Build history of the part. All positions in model axes, mm. A direction names the side the tool comes from. Round coordinates to 2 decimals unless told otherwise and drop trailing zeros. Write each loop counter-clockwise with the first axis right and the second up, starting at its lowest first coordinate (ties: lowest second). Pieces come first, ordered by that corner, then holes. Notation, with made-up numbers: (39, 25) -> (98, 25) arc R7 cw to (98, 29) -> close; hole circle Ø9 at (66.5, 13). An arc over 180 degrees is marked (long way). One line per question, with ' | ' between items.
from build123d import *

# Parameters (mm, degrees)
SKETCH002_R     = 6.5
SKETCH002_R_2   = 3
PAD_DEPTH       = 8
SKETCH003_R     = 7.7
POCKET_DEPTH    = 2
SKETCH004_R     = 3
POCKET001_DEPTH = 31
SKETCH005_R     = 2
PAD001_DEPTH    = 2


with BuildPart() as part:
    # Sketch002 → Pad (new body)
    with BuildSketch(Plane.XZ):
        with BuildLine():
            Line((-6.339746, 5), (6.339746, 5))
            ThreePointArc((25, 0), (17.58819, 9.659258), (6.339746, 5))
            Line((25, -14.5), (25, 0))
            Line((15, -14.5), (25, -14.5))
            Line((15, -10), (15, -14.5))
            ThreePointArc((6.339746, -5), (10, -8.660254), (15, -10))
            Line((-6.339746, -5), (6.339746, -5))
            ThreePointArc((-15, -10), (-10, -8.660254), (-6.339746, -5))
            Line((-15, -10), (-15, -14.5))
            Line((-25, -14.5), (-15, -14.5))
            Line((-25, 0), (-25, -14.5))
            ThreePointArc((-6.339746, 5), (-17.58819, 9.659258), (-25, 0))
        make_face()
        with Locations((-15, 0)):
            Circle(SKETCH002_R, mode=Mode.SUBTRACT)
        with Locations((15, 0)):
            Circle(SKETCH002_R, mode=Mode.SUBTRACT)
        Circle(SKETCH002_R_2, mode=Mode.SUBTRACT)
    extrude(amount=PAD_DEPTH)

    # Sketch003 (on Face16 of Pad) → Pocket (cut)
    with BuildSketch(Plane(origin=(0, 0, 0), x_dir=(1, 0, 0), z_dir=(0, 1, 0))):
        with Locations((-15, 0)):
            Circle(SKETCH003_R)
        with Locations((15, 0)):
            Circle(SKETCH003_R)
    extrude(amount=-POCKET_DEPTH, mode=Mode.SUBTRACT)

    # Sketch004 → Pocket001 (cut, symmetric)
    with BuildSketch(Plane.YZ):
        with Locations((-4, -10)):
            Circle(SKETCH004_R)
    extrude(amount=POCKET001_DEPTH, both=True, mode=Mode.SUBTRACT)

    # Sketch005 → Pad001 (join)
    with BuildSketch(Plane.XY.offset(-14.5)):
        with BuildLine():
            Line((-25, 0), (-15, 0))
            Line((-15, 0), (-15, 3.5))
            ThreePointArc((-15, 3.5), (-20, 8.5), (-25, 3.5))
            Line((-25, 0), (-25, 3.5))
        make_face()
        with Locations((-20, 3.5)):
            Circle(SKETCH005_R, mode=Mode.SUBTRACT)
        with BuildLine():
            Line((15, 0), (25, 0))
            Line((25, 0), (25, 3.5))
            ThreePointArc((25, 3.5), (20, 8.5), (15, 3.5))
            Line((15, 0), (15, 3.5))
        make_face()
        with Locations((20, 3.5)):
            Circle(SKETCH005_R, mode=Mode.SUBTRACT)
    extrude(amount=PAD001_DEPTH)


solid = part.part
(1) Mould opens along Z. For faces 1 (the flat face through (12, -2, 6)), 2 (the flat face through (20, 0, -14.5)), 3 (the cylindrical face through (18.002, 3.588, -13.514)) say: pulls with the +Z half, pulls with the -Z half, needs draft (parallel to the pull), parting line crosses it, or undercut.
Calculated:
face 1: undercut | face 2: pulls with the -Z half | face 3: needs draft
(2) 3-axis set-ups, long thin cutter, end or side, ignore diameter. For faces 4 (the cylindrical face through (-7, -4, -6)), 5 (the flat face through (18.8, 5.3, -12.5)), 6 (the flat face through (-18, -2, 6)), 7 (the flat face through (0, -4, 5)): which of +Z, -Z, +X, -X, +Y, -Y reach the whole face in a straight line?
Calculated:
face 4: -Z, +Y, -Y | face 5: +Z, +X, -X, +Y | face 6: +Y | face 7: +Z, +Y, -Y
(3) Wall check: line 1 (Y direction, x = -19.75, z = -10); line 2 (Y direction, x = -20, z = -13.45); line 3 (Z direction, x = -15.5, y = -4). Give the ranges that are in metal, low to high. Write a range as from..to.
Calculated:
line 1: -8..-7, -1..0 | line 2: -8..1.5, 5.5..8.5 | line 3: -14.5..-13, -7..-6.48, 6.48..9.99
(4) Drop flat-ended pins along their axis: pin 1 (12.5 mm diameter, centred on x = -12.5, z = 0, fed in from +Y); pin 2 (9.5 mm diameter, centred on x = 21.5, y = 4, fed in from +Z); pin 3 (8 mm diameter, centred on y = -4, z = -10, fed in from -X); pin 4 (4 mm diameter, centred on x = -1, y = -2, fed in from +Z). Give the stop position or say it passes through.
Calculated:
pin 1: y = 0 | pin 2: z = 9.19 | pin 3: x = -25 | pin 4: z = 5
(5) Slice it at C-C (y = -4.25). Write the cut outline in (x, z), then the cut area to 3 significant figures.
Calculated:
outline: (-25, -14.5) -> (-15, -14.5) -> (-15, -12.99) -> (-25, -12.99) -> close; (-25, -7.01) -> (-7.87, -7.01) arc R10 ccw to (-6.34, -5) -> (6.34, -5) arc R10 ccw to (7.87, -7.01) -> (25, -7.01) -> (25, 0) arc R10 ccw to (6.34, 5) -> (-6.34, 5) arc R10 ccw to (-25, 0) -> close; (15, -14.5) -> (25, -14.5) -> (25, -12.99) -> (15, -12.99) -> close; hole circle Ø13 at (-15, 0); hole circle Ø6 at (0, 0); hole circle Ø13 at (15, 0) | area: 427 mm2
(6) Slice it at D-D (y = 4.25). Write the cut outline in (x, z).
Calculated:
outline: (-24.94, -14.5) -> (-21.85, -14.5) -> (-21.85, -12.5) -> (-24.94, -12.5) -> close; (-18.15, -14.5) -> (-15.06, -14.5) -> (-15.06, -12.5) -> (-18.15, -12.5) -> close; (15.06, -14.5) -> (18.15, -14.5) -> (18.15, -12.5) -> (15.06, -12.5) -> close; (21.85, -14.5) -> (24.94, -14.5) -> (24.94, -12.5) -> (21.85, -12.5) -> close
(7) Slice it at A-A (x = -17.5). Write the cut outline in (y, z).
Calculated:
outline: (-8, -14.5) -> (7.83, -14.5) -> (7.83, -12.5) -> (0, -12.5) -> (0, -7.28) -> (-2, -7.28) -> (-2, -6) -> (-8, -6) -> close; (-8, 6) -> (-2, 6) -> (-2, 7.28) -> (0, 7.28) -> (0, 9.68) -> (-8, 9.68) -> close; hole circle Ø6 at (-4, -10)
(8) Slice it at B-B (x = 20). Write the cut outline in (y, z), then the cut area to 3 significant figures.
Calculated:
outline: (-8, -14.5) -> (1.5, -14.5) -> (1.5, -12.5) -> (0, -12.5) -> (0, -5.86) -> (-2, -5.86) -> (-2, -4.15) -> (-8, -4.15) -> close; (-8, 4.15) -> (-2, 4.15) -> (-2, 5.86) -> (0, 5.86) -> (0, 8.66) -> (-8, 8.66) -> close; (5.5, -14.5) -> (8.5, -14.5) -> (8.5, -12.5) -> (5.5, -12.5) -> close; hole circle Ø6 at (-4, -10) | area: 92.7 mm2
